```python
from build123d import *

# Parameters (mm, degrees)
SKETCH_1_W      = 12
SKETCH_1_H      = 70
SKETCH_1_H_2    = 10
EXTRUDE_1_DEPTH = 140


with BuildPart() as part:
    # Эскиз1 → Бобышка-Вытянуть1 (new, symmetric)
    with BuildSketch(Plane.XY):
        Polygon((-33, 35), (-6, 35), (6, 35), (33, 35), (45, 35), (45, 47), (-45, 47), (-45, 35), align=None)
        Rectangle(SKETCH_1_W, SKETCH_1_H)
        Polygon((6, -35), (-6, -35), (-50, -35), (-50, -47), (50, -47), (50, -35), align=None)
        with Locations((39, 30)):
            Rectangle(SKETCH_1_W, SKETCH_1_H_2)
        with Locations((-39, 30)):
            Rectangle(SKETCH_1_W, SKETCH_1_H_2)
    extrude(amount=EXTRUDE_1_DEPTH, both=True)


solid = part.part
```
Part model, mm, in its own coordinate system. A direction names the side the tool comes from. Give positions to 0.01 mm unless a question says otherwise; leave off trailing zeros. Write each loop counter-clockwise with the first axis right and the second up, starting at its lowest first coordinate (ties: lowest second). Pieces come first, ordered by that corner, then holes. Notation, with made-up numbers: (-40, 30.25) -> (1, 30.25) arc R14 ccw to (1, 41.25) -> close; hole circle Ø4 at (-5, 9). An arc over 180 degrees is marked (long way). Put each result on its own line as item: value. Start each with the question number.
Item 1: Pull direction Y, two halves, no side cores. Call faces 6 (the face through (-1, -47, 2)), 7 (the face through (28, -35, 2)), 8 (the face through (19, 35, 2)), 9 (the face through (0, 4, -140)): pulls with the +Y half, pulls with the -Y half, needs draft (parallel to the pull), parting line crosses it, or undercut.
Item 2: Cut at B-B (y = 28.5). List the corners of the cut face in (x, z).
Item 3: Pin check, flat tips, straight feed: pin 1 Ø3 at (x, y) = (9, 17.5) entering from +Z; pin 2 Ø5 at (y, z) = (-32, -79.5) entering from -X; pin 3 Ø6.5 at (y, z) = (38, 19) entering from -X; pin 4 Ø1.5 at (y, z) = (17.5, 65) entering from +X. Stop position of each tip, or through.
Item 4: Wall check: L1, parallel to X at y = 30.5, z = 66; L2, parallel to Y at x = 32.5, z = 29; L3, parallel to Y at x = 40, z = 75. Give the ranges that are in metal, low to high. Write a range as [from, to].
Item 5: Cut at C-C (z = 16.5). List the corners of the cut face in (x, y), then the cut area to 3 significant figures.
Item 6: Which spindle directions (+Z, -Z, +X, -X, +Y, -Y) get a long thin tool onto all of the face, cutting with end or side? Do faces 1 (the face through (-20, 35, 2)), 2 (the face through (-45, 36, 2)), 3 (the face through (-39, 25, 2)), 4 (the face through (45, 36, 2)), 5 (the face through (39, 25, 2)). Say none if no direction does.
Item 7: Cut at D-D (x = -19). List the corners of the cut face in (y, z), then the cut area to 3 significant figures.
Item 8: Cut at A-A (x = -38). List the corners of the cut face in (y, z), then the cut area to 3 significant figures.
Answer list:
1. face 6: pulls with the -Y half
1. face 7: undercut
1. face 8: undercut
1. face 9: needs draft
2. outline: (-45, -140) -> (-33, -140) -> (-33, 140) -> (-45, 140) -> close; (-6, -140) -> (6, -140) -> (6, 140) -> (-6, 140) -> close; (33, -140) -> (45, -140) -> (45, 140) -> (33, 140) -> close
3. pin 1: passes through
3. pin 2: stops at x = -6
3. pin 3: stops at x = -45
3. pin 4: stops at x = 6
4. L1: x = [-45, -33], [-6, 6], [33, 45]
4. L2: y = [-47, -35], [35, 47]
4. L3: y = [-47, -35], [25, 47]
5. outline: (-50, -47) -> (50, -47) -> (50, -35) -> (6, -35) -> (6, 35) -> (33, 35) -> (33, 25) -> (45, 25) -> (45, 47) -> (-45, 47) -> (-45, 25) -> (-33, 25) -> (-33, 35) -> (-6, 35) -> (-6, -35) -> (-50, -35) -> close
5. area: 3,360 mm2
6. face 1: +Z, -Z
6. face 2: +Z, -Z, -X, +Y
6. face 3: +Z, -Z, -X
6. face 4: +Z, -Z, +X, +Y
6. face 5: +Z, -Z, +X
7. outline: (-47, -140) -> (-35, -140) -> (-35, 140) -> (-47, 140) -> close; (35, -140) -> (47, -140) -> (47, 140) -> (35, 140) -> close
7. area: 6,720 mm2
8. outline: (-47, -140) -> (-35, -140) -> (-35, 140) -> (-47, 140) -> close; (25, -140) -> (47, -140) -> (47, 140) -> (25, 140) -> close
8. area: 9,520 mm2
